Model file for the job. Use its own axes, mm. Face numbers are marked on the shaded views. A direction names the side the tool comes from. Give positions to 0.01 mm unless a question says otherwise; leave off trailing zeros. Write each loop counter-clockwise with the first axis right and the second up, starting at its lowest first coordinate (ties: lowest second). Pieces come first, ordered by that corner, then holes. Notation, with made-up numbers: (28.5, 77) - (80.5, 77) arc R19 ccw to (80.5, 98) - close; hole circle Ø4 at (16.5, 83.25). An arc over 180 degrees is marked (long way). One line per item, written item: value. Start each with the question number.
(1) Cut at A-A, the plane z = 128.8. List the corners of the cut face in (x, y), and give its area (3 significant figures).
(2) Cut at D-D, the plane y = 33. List the corners of the cut face in (x, z).
(3) Probe L1, parallel to Y at x = -8.5, z = 83; L2, parallel to Z at x = 2, y = 6. List the from-to ranges inside material, lowest first.
(4) Drop flat-ended pins along their axis: P1, Ø5.5, axis at x = 16, y = 73.6, coming from the +Z side; P2, Ø1.5, axis at x = -5.5, z = 38, coming from the +Y side. Give the stop position or say it passes through.
(5) Cut at B-B, the plane x = 0. List the corners of the cut face in (y, z).
(6) Cut at C-C, the plane x = -10.5. List the corners of the cut face in (y, z), and give its area (3 significant figures).
(7) 3-axis set-ups, long thin cutter, end or side, ignore diameter. For the marked faces 1 and 2: which of +Z, -Z, +X, -X, +Y, -Y reach the whole face in a straight line?
from build123d import *

# Parameters (mm, degrees)
SKETCH1_W              = 44
SKETCH1_H              = 360
BASE_FLANGE1_DEPTH     = 1.2
SKETCHED_START         = -22
SKETCHED_BEND1_DEPTH   = 44
SKETCHED_BEND1_2_DEPTH = 44
SKETCH7_R              = 2.205641569
CUT_EXTRUDE1_DEPTH     = 10
SKETCH8_R              = 4
CUT_EXTRUDE2_DEPTH     = 10


# Read off the part's stored shape, not the designer's step: Sketched Bend1
# Sheet-metal steps are written as plain solids
with BuildPart() as part:
    # Sketch1 → Base-Flange1 (new body)
    with BuildSketch(Plane(origin=(0, 0, 0), x_dir=(1, 0, 0), z_dir=(0, 1, 0))):
        Rectangle(SKETCH1_W, SKETCH1_H)
    extrude(amount=-BASE_FLANGE1_DEPTH)

    # Sketched Bend1 outline → Sketched Bend1 (cut)
    with BuildSketch(Plane.YZ.offset(SKETCHED_START)):
        with BuildLine():
            Line((0, -180), (0, -85.054444388))
            ThreePointArc((0, -85.054444388), (-0.872269031, -84.341342484), (-1.2, -83.2634))
            Line((-1.2, -83.2634), (-1.2, -180))
            Line((-1.2, -180), (0, -180))
        make_face()
    extrude(amount=SKETCHED_BEND1_DEPTH, mode=Mode.SUBTRACT)

    # Sketched Bend1 2 outline → Sketched Bend1 2 (add)
    with BuildSketch(Plane.YZ.offset(SKETCHED_START)):
        with BuildLine():
            Line((93.6, -84), (0.7366, -84))
            ThreePointArc((0.7366, -84), (0.215745145, -83.784254855), (0, -83.2634))
            Line((0, -83.2634), (0, -85.054444388))
            ThreePointArc((0, -85.054444388), (0.361178238, -85.163262642), (0.7366, -85.2))
            Line((0.7366, -85.2), (93.6, -85.2))
            Line((93.6, -85.2), (93.6, -84))
        make_face()
    extrude(amount=SKETCHED_BEND1_2_DEPTH)

    # Sketch7 → Cut-Extrude1 (cut)
    with BuildSketch(Plane(origin=(0, 0, -85.2), x_dir=(-1, 0, 0), z_dir=(0, 0, -1))):
        with Locations(Location((-16, 73.6, 0), (0, 0, 90))):
            Circle(SKETCH7_R)
        with Locations(Location((16, 73.6, 0), (0, 0, 90))):
            Circle(SKETCH7_R)
    extrude(amount=-CUT_EXTRUDE1_DEPTH, mode=Mode.SUBTRACT)

    # Sketch8 → Cut-Extrude2 (cut)
    with BuildSketch(Plane.XZ.offset(1.2)):
        with Locations(Location((0, -11.2, 0), (0, 0, 270))):
            Circle(SKETCH8_R)
        with Locations(Location((0, 128.8, 0), (0, 0, 270))):
            Circle(SKETCH8_R)
    extrude(amount=-CUT_EXTRUDE2_DEPTH, mode=Mode.SUBTRACT)


solid = part.part
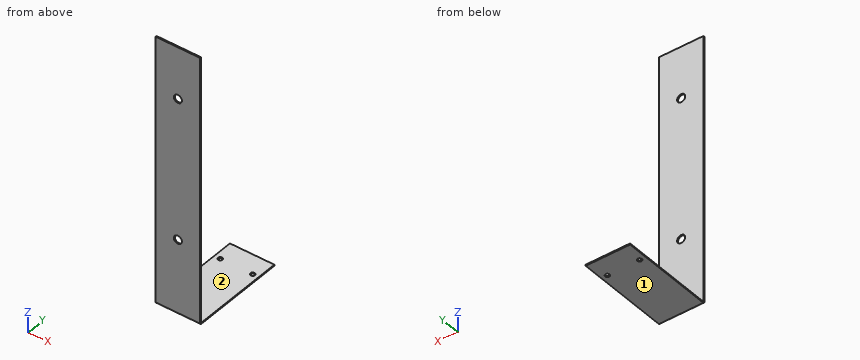
Answers follow:
1. outline: (-22, -1.2) - (-4, -1.2) - (-4, 0) - (-22, 0) - close; (4, -1.2) - (22, -1.2) - (22, 0) - (4, 0) - close
1. area: 43.2 mm²
2. outline: (-22, -85.2) - (22, -85.2) - (22, -84) - (-22, -84) - close
3. L1: y = -1.2 to 0
3. L2: z = -85.2 to -84
4. P1: stops at z = -84
4. P2: stops at y = 0
5. outline: (-1.2, -83.26) arc R1.94 ccw to (0.74, -85.2) - (93.6, -85.2) - (93.6, -84) - (0.74, -84) arc R0.74 cw to (0, -83.26) - (0, -15.2) - (-1.2, -15.2) - close; (-1.2, -7.2) - (0, -7.2) - (0, 124.8) - (-1.2, 124.8) - close; (-1.2, 132.8) - (0, 132.8) - (0, 180) - (-1.2, 180) - close
6. outline: (-1.2, -83.26) arc R1.94 ccw to (0.74, -85.2) - (93.6, -85.2) - (93.6, -84) - (0.74, -84) arc R0.74 cw to (0, -83.26) - (0, 180) - (-1.2, 180) - close
6. area: 430 mm²
7. face 1: -Z, +X, -X, +Y, -Y
7. face 2: +Z, +X, -X, +Y
